from build123d import *

# Parameters (mm, degrees)
SKETCH1_R           = 3.25
SKETCH1_R_2         = 10.5
BOSS_EXTRUDE1_DEPTH = 8.73125
SKETCH2_R           = 12.05
CUT_EXTRUDE1_DEPTH  = 6.35
SKETCH6_R           = 1.7
CUT_EXTRUDE4_DEPTH  = 189.881536225
FILLET1_R           = 2


with BuildPart() as part:
    # Sketch1 → Boss-Extrude1 (new body)
    with BuildSketch(Plane(origin=(0, 0, 0), x_dir=(1, 0, 0), z_dir=(0, 1, 0))):
        with BuildLine():
            Line((-110, -100), (0, -100))
            Line((0, -100), (0, 0))
            Line((0, 0), (-110, 0))
            ThreePointArc((-110, 0), (-160, -50), (-110, -100))
        make_face()
        with Locations(Location((-13, -10, 0), (0, 0, 270))):
            Circle(SKETCH1_R, mode=Mode.SUBTRACT)
        with Locations(Location((-37, -10, 0), (0, 0, 270))):
            Circle(SKETCH1_R, mode=Mode.SUBTRACT)
        with Locations(Location((-18, -50, 0), (0, 0, 270))):
            Circle(SKETCH1_R, mode=Mode.SUBTRACT)
        with Locations(Location((-13, -90, 0), (0, 0, 270))):
            Circle(SKETCH1_R, mode=Mode.SUBTRACT)
        with Locations(Location((-37, -90, 0), (0, 0, 270))):
            Circle(SKETCH1_R, mode=Mode.SUBTRACT)
        with Locations(Location((-42, -50, 0), (0, 0, 270))):
            Circle(SKETCH1_R, mode=Mode.SUBTRACT)
        with Locations(Location((-110, -50, 0), (0, 0, 270))):
            Circle(SKETCH1_R_2, mode=Mode.SUBTRACT)
    extrude(amount=BOSS_EXTRUDE1_DEPTH)

    # Sketch2 → Cut-Extrude1 (cut)
    with BuildSketch(Plane(origin=(0, 8.73125, 0), x_dir=(1, 0, 0), z_dir=(0, 1, 0))):
        with Locations(Location((-110, -50, 0), (0, 0, 270))):
            Circle(SKETCH2_R)
    extrude(amount=-CUT_EXTRUDE1_DEPTH, mode=Mode.SUBTRACT)

    # Sketch6 → Cut-Extrude4 (cut, through all)
    with BuildSketch(Plane(origin=(0, 8.73125, 0), x_dir=(1, 0, 0), z_dir=(0, 1, 0))):
        with Locations(Location((-147, -50, 0), (0, 0, 270))):
            Circle(SKETCH6_R)
        with BuildLine():
            Line((-133.793921789, -41.071004616), (-145.477766874, -38.051775556))
            ThreePointArc((-145.477766874, -38.051775556), (-133.72851482, -21.93564785), (-115.86984126, -13.056330604))
            Line((-115.86984126, -13.056330604), (-112.417796121, -25.271259557))
            ThreePointArc((-112.417796121, -25.271259557), (-125.525564083, -29.897413384), (-133.793921789, -41.071004616))
        make_face()
        with BuildLine():
            Line((-105.513705843, -25.271259557), (-104.258758681, -12.795366162))
            Line((-104.258758681, -12.795366162), (-53.734606151, -12.795366162))
            ThreePointArc((-53.734606151, -12.795366162), (-41.801024618, -26.273023002), (-24.46272378, -21.431439979))
            ThreePointArc((-24.46272378, -21.431439979), (-19.304766449, -24.941567185), (-13.556215286, -27.366371581))
            Line((-13.556215286, -27.366371581), (-13.556215286, -33.028900538))
            ThreePointArc((-13.556215286, -33.028900538), (-22.279595055, -34.31177696), (-30.264301501, -38.051775556))
            ThreePointArc((-30.264301501, -38.051775556), (-45.81064331, -34.0967888), (-59.032653211, -43.180241783))
            Line((-59.032653211, -43.180241783), (-84.662721734, -41.071004616))
            ThreePointArc((-84.662721734, -41.071004616), (-93.117084888, -30.569825722), (-105.513705843, -25.271259557))
        make_face()
        with BuildLine():
            Line((-115.86984126, -86.943669396), (-112.417796121, -74.728740443))
            ThreePointArc((-112.417796121, -74.728740443), (-125.525564083, -70.102586616), (-133.793921789, -58.928995384))
            Line((-133.793921789, -58.928995384), (-145.477766874, -61.948224444))
            ThreePointArc((-145.477766874, -61.948224444), (-133.72851482, -78.06435215), (-115.86984126, -86.943669396))
        make_face()
        with BuildLine():
            Line((-104.258758681, -87.204633838), (-53.734606151, -87.204633838))
            ThreePointArc((-53.734606151, -87.204633838), (-41.801024618, -73.726976998), (-24.46272378, -78.568560021))
            ThreePointArc((-24.46272378, -78.568560021), (-19.304766449, -75.058432815), (-13.556215286, -72.633628419))
            Line((-13.556215286, -72.633628419), (-13.556215286, -66.971099462))
            ThreePointArc((-13.556215286, -66.971099462), (-22.279595055, -65.68822304), (-30.264301501, -61.948224444))
            ThreePointArc((-30.264301501, -61.948224444), (-45.81064331, -65.9032112), (-59.032653211, -56.819758217))
            Line((-59.032653211, -56.819758217), (-84.662721734, -58.928995384))
            ThreePointArc((-84.662721734, -58.928995384), (-93.117084888, -69.430174278), (-105.513705843, -74.728740443))
            Line((-105.513705843, -74.728740443), (-104.258758681, -87.204633838))
        make_face()
    extrude(amount=-CUT_EXTRUDE4_DEPTH, mode=Mode.SUBTRACT)

    # Fillet1
    fillet1_edges = [part.edges().sort_by_distance(p)[0] for p in [
        (-13.556215286, 4.365625, 33.028900538),
        (-30.264301501, 4.365625, 38.051775556),
        (-59.032653211, 4.365625, 43.180241783),
        (-112.417796121, 4.365625, 25.271259557),
        (-133.793921789, 4.365625, 41.071004616),
        (-145.477766874, 4.365625, 38.051775556),
        (-115.86984126, 4.365625, 13.056330604),
        (-24.46272378, 4.365625, 78.568560021),
        (-53.734606151, 4.365625, 87.204633838),
        (-104.258758681, 4.365625, 87.204633838),
        (-105.513705843, 4.365625, 74.728740443),
        (-84.662721734, 4.365625, 58.928995384),
        (-59.032653211, 4.365625, 56.819758217),
        (-30.264301501, 4.365625, 61.948224444),
        (-13.556215286, 4.365625, 66.971099462),
        (-13.556215286, 4.365625, 72.633628419),
        (-115.86984126, 4.365625, 86.943669396),
        (-145.477766874, 4.365625, 61.948224444),
        (-133.793921789, 4.365625, 58.928995384),
        (-112.417796121, 4.365625, 74.728740443),
        (-84.662721734, 4.365625, 41.071004616),
        (-105.513705843, 4.365625, 25.271259557),
        (-104.258758681, 4.365625, 12.795366162),
        (-53.734606151, 4.365625, 12.795366162),
        (-24.46272378, 4.365625, 21.431439979),
        (-13.556215286, 4.365625, 27.366371581),
    ]]
    fillet(fillet1_edges, radius=FILLET1_R)


solid = part.part
Build history of the part. All positions in model axes, mm. A direction names the side the tool comes from. Coordinates: 2 decimals unless noted, no trailing zeros. Write each loop counter-clockwise with the first axis right and the second up, starting at its lowest first coordinate (ties: lowest second). Pieces come first, ordered by that corner, then holes.
(1) Mould opens along Z. For faces 4 (the cylindrical face through (-92.72, 4.427, 69.123)), 5 (the cylindrical face through (-159.988, 4.305, 48.901)), 6 (the cylindrical face through (-116.39, 1.17, 41.67)), 7 (the flat face through (0, 4, 51)) say: pulls with the +Z half, pulls with the -Z half, needs draft (parallel to the pull), parting line crosses it, or undercut.
(2) Cut at D-D on y = 6.5. State how many separate pieces and enclosed holes the cut face has, and give its area (3 significant figures).
(3) Cut at B-B on x = -80. List the corners of the cut face in (y, z), and give its area (3 significant figures).
(4) Cut at C-C on x = -147. List the corners of the cut face in (y, z), and give its area (3 significant figures).
(5) Pin check, flat tips, straight feed: pin 1 Ø19.5 at (x, z) = (-110, 50) entering from +Y; pin 2 Ø12 at (x, z) = (-31.5, 45) entering from -Y; pin 3 Ø2.5 at (y, z) = (3.5, 29.5) entering from -X; pin 4 Ø1.5 at (y, z) = (7.5, 45.5) entering from -X. Stop position of each tip, or through.
(6) Cut at A-A on x = -42. List the corners of the cut face in (y, z).
(7) 3-axis set-ups, long thin cutter, end or side, ignore diameter. For faces 1 (the flat face through (-63, 0, 49)), 2 (the cylindrical face through (-42.1, 4.43, 73.82)), 3 (the flat face through (-100, 2.381, 46)): which of +Z, -Z, +X, -X, +Y, -Y reach the whole face in a straight line?
(8) Drill centre lines: line 1 (X direction, y = 4.75, z = 92.5); line 2 (X direction, y = 4.75, z = 21); line 3 (X direction, y = 1.25, z = 13). Where is each one in solid material? Low to high.
Working result:
1. face 4: undercut
1. face 5: parting line crosses it
1. face 6: undercut
1. face 7: needs draft
2. separate pieces: 1
2. enclosed holes: 12
2. area: 10,100 mm2
3. outline: (0, 0) - (8.73, 0) - (8.73, 12.8) - (0, 12.8) - close; (0, 41.45) - (8.73, 41.45) - (8.73, 58.55) - (0, 58.55) - close; (0, 87.2) - (8.73, 87.2) - (8.73, 100) - (0, 100) - close
3. area: 373 mm2
4. outline: (0, 16.37) - (8.73, 16.37) - (8.73, 48.3) - (0, 48.3) - close; (0, 51.7) - (8.73, 51.7) - (8.73, 83.63) - (0, 83.63) - close
4. area: 558 mm2
5. pin 1: passes through
5. pin 2: stops at y = 0
5. pin 3: stops at x = -156.15
5. pin 4: stops at x = -159.86
6. outline: (0, 0) - (8.73, 0) - (8.73, 26.21) - (0, 26.21) - close; (0, 33.8) - (8.73, 33.8) - (8.73, 46.75) - (0, 46.75) - close; (0, 53.25) - (8.73, 53.25) - (8.73, 66.2) - (0, 66.2) - close; (0, 73.79) - (8.73, 73.79) - (8.73, 100) - (0, 100) - close
7. face 1: +Z, -Z, +X, -X, -Y
7. face 2: +Y, -Y
7. face 3: +Y
8. line 1: x = -136.34 to -39.08, -34.92 to -15.08, -10.92 to 0
8. line 2: x = -150.73 to -132.58, -113.62 to -105.08, -49.92 to 0
8. line 3: x = -143.63 to -103.33, -54.47 to -38.25, -35.75 to -14.25, -11.75 to 0
